from build123d import *

# Parameters (mm, degrees)
SKETCH1_W                = 42
SKETCH1_H                = 120
SKETCH1_R                = 7.5
BOSS_EXTRUDE1_DEPTH      = 10
BOSS_EXTRUDE2_DEPTH      = 6
BOSS_EXTRUDE3_DEPTH      = 6
BOSS_EXTRUDE3_DEPTH_BACK = 42
BOSS_EXTRUDE4_START      = 36
BOSS_EXTRUDE4_DEPTH      = 36
BOSS_EXTRUDE7_START      = -25
SKETCH5_R                = 6
BOSS_EXTRUDE7_DEPTH      = 70
CUT_EXTRUDE1_START       = -70
CUT_EXTRUDE1_DEPTH       = 70


with BuildPart() as part:
    # Sketch1 → Boss-Extrude1 (new body)
    with BuildSketch(Plane(origin=(0, 0, 0), x_dir=(1, 0, 0), z_dir=(0, 1, 0))):
        with Locations((21, 60)):
            Rectangle(SKETCH1_W, SKETCH1_H)
        with Locations(Location((21, 15, 0), (0, 0, 270))):
            Circle(SKETCH1_R, mode=Mode.SUBTRACT)
        with Locations(Location((21, 105, 0), (0, 0, 90))):
            Circle(SKETCH1_R, mode=Mode.SUBTRACT)
    extrude(amount=BOSS_EXTRUDE1_DEPTH)

    # Sketch2 → Boss-Extrude2 (add)
    with BuildSketch(Plane(origin=(42, 0, 0), x_dir=(0, 0, -1), z_dir=(1, 0, 0))):
        with BuildLine():
            Line((90, 25), (90, 86.972243623))
            ThreePointArc((90, 86.972243623), (60, 70), (30, 86.972243623))
            Line((30, 86.972243623), (30, 25))
            ThreePointArc((30, 25), (25.606601718, 14.393398282), (15, 10))
            Line((15, 10), (105, 10))
            ThreePointArc((105, 10), (94.393398282, 14.393398282), (90, 25))
        make_face()
    extrude(amount=-BOSS_EXTRUDE2_DEPTH)

    # Sketch3 → Boss-Extrude3 (add, two sides: drawn at the far end of the back side and taken through both)
    with BuildSketch(Plane(origin=(42, 0, 0), x_dir=(0, 0, -1), z_dir=(1, 0, 0)).offset(-BOSS_EXTRUDE3_DEPTH_BACK)):
        with BuildLine():
            Line((61.5, 134.962476533), (61.5, 139.96784237))
            ThreePointArc((61.5, 139.96784237), (60, 70), (58.5, 139.96784237))
            Line((58.5, 139.96784237), (58.5, 134.962476533))
            ThreePointArc((58.5, 134.962476533), (60, 75), (61.5, 134.962476533))
        make_face()
    extrude(amount=BOSS_EXTRUDE3_DEPTH + BOSS_EXTRUDE3_DEPTH_BACK)

    # Sketch4 → Boss-Extrude4 (add)
    with BuildSketch(Plane.ZY.offset(-36).offset(BOSS_EXTRUDE4_START)):
        with BuildLine():
            Line((-61.5, 10), (-58.5, 10))
            Line((-58.5, 10), (-58.5, 70.03215763))
            ThreePointArc((-58.5, 70.03215763), (-60, 70), (-61.5, 70.03215763))
            Line((-61.5, 70.03215763), (-61.5, 10))
        make_face()
    extrude(amount=-BOSS_EXTRUDE4_DEPTH)

    # Sketch5 → Boss-Extrude7 (add)
    with BuildSketch(Plane.XY.offset(BOSS_EXTRUDE7_START)):
        with BuildLine():
            Line((7, 105), (35, 105))
            Line((35, 105), (35, 147))
            ThreePointArc((35, 147), (21, 161), (7, 147))
            Line((7, 147), (7, 105))
        make_face()
        with Locations((21, 147)):
            Circle(SKETCH5_R, mode=Mode.SUBTRACT)
    extrude(amount=-BOSS_EXTRUDE7_DEPTH)

    # Sketch6 → Cut-Extrude1 (cut)
    with BuildSketch(Plane(origin=(48, 0, 0), x_dir=(0, 0, -1), z_dir=(1, 0, 0)).offset(CUT_EXTRUDE1_START)):
        with BuildLine():
            Line((58.5, 139.96784237), (58.5, 134.962476533))
            ThreePointArc((58.5, 134.962476533), (60, 75), (61.5, 134.962476533))
            Line((61.5, 134.962476533), (61.5, 139.96784237))
            ThreePointArc((61.5, 139.96784237), (60, 140), (58.5, 139.96784237))
        make_face()
    extrude(amount=CUT_EXTRUDE1_DEPTH, mode=Mode.SUBTRACT)


solid = part.part
Geometry: final body of the model. Coordinates: model frame, mm. A direction names the side the tool comes from. Round coordinates to 2 decimals unless told otherwise and drop trailing zeros. Loops run counter-clockwise (first coordinate to the right, second up) from the corner with the lowest first, then second, coordinate; pieces in that order, holes last. Notation, with made-up numbers: (-30.5, 40) -> (-21.5, 40) arc R35 cw to (-21.5, 79) -> close; hole circle Ø1 at (12, -36.5). An arc over 180 degrees is marked (long way). One line per question, with ' | ' between items. Start each with the question number.
1. Mould query, pull axis Z, two halves, no side actions, for faces 1 (the face through (21, 10, -30)), 2 (the face through (24, 138, -58.5)), 3 (the face through (21, 5, 0)). Classes: pulls with the +Z half, pulls with the -Z half, needs draft (parallel to the pull), parting line crosses it, or undercut.
2. Contact query for flat-ended pins moving along their axis: pin 1 (3 mm diameter, centred on x = 39.5, y = 55.5, fed in from +Z); pin 2 (10 mm diameter, centred on y = 29.5, z = -62.5, fed in from +X); pin 3 (8 mm diameter, centred on x = 25.5, y = 107, fed in from -Z). Output: stop coordinate, or through.
3. Section B-B on y = 149.5. Output: boundary loops of the cut face in (x, z), and give its area (3 significant figures).
4. Section C-C on y = 37.5. Output: boundary loops of the cut face in (x, z), and give its area (3 significant figures).
5. Section D-D on y = 122. Output: boundary loops of the cut face in (x, z), and give its area (3 significant figures).
6. Section A-A on x = 21. Output: boundary loops of the cut face in (y, z).
7. Line query: line 1 along X through (y, z) = (7, -15); line 2 along Z through (x, y) = (20, 105); line 3 along Y through (x, z) = (2, -34.5). Output: solid intervals per line, ascending. Write a range as [from, to].
8. Set-up query: faces 4 (the face through (39, 56, -90)), 5 (the face through (18, 40, -58.5)), 6 (the face through (24, 137, -61.5)). Return all of +Z, -Z, +X, -X, +Y, -Y with unobstructed straight access to the full face (end or side cutting, diameter ignored); none if empty.
Returned:
1) face 1: needs draft | face 2: undercut | face 3: pulls with the +Z half
2) pin 1: stops at z = -30 | pin 2: stops at x = 42 | pin 3: stops at z = -95
3) outline: (7.23, -95) -> (15.55, -95) -> (15.55, -25) -> (7.23, -25) -> close; (26.45, -95) -> (34.77, -95) -> (34.77, -25) -> (26.45, -25) -> close | area: 1,160 mm2
4) outline: (0, -61.5) -> (36, -61.5) -> (36, -90) -> (42, -90) -> (42, -30) -> (36, -30) -> (36, -58.5) -> (0, -58.5) -> close | area: 468 mm2
5) outline: (0, -90.59) -> (7, -90.59) -> (7, -95) -> (35, -95) -> (35, -90.59) -> (48, -90.59) -> (48, -84.72) -> (0, -84.72) -> close; (0, -35.28) -> (48, -35.28) -> (48, -29.41) -> (35, -29.41) -> (35, -25) -> (7, -25) -> (7, -29.41) -> (0, -29.41) -> close | area: 811 mm2
6) outline: (0, -120) -> (10, -120) -> (10, -112.5) -> (0, -112.5) -> close; (0, -97.5) -> (10, -97.5) -> (10, -61.5) -> (70.03, -61.5) arc R35 ccw to (105, -95) -> (141, -95) -> (141, -25) -> (105, -25) arc R35 ccw to (70.03, -58.5) -> (10, -58.5) -> (10, -22.5) -> (0, -22.5) -> close; (0, -7.5) -> (10, -7.5) -> (10, 0) -> (0, 0) -> close; (153, -95) -> (161, -95) -> (161, -25) -> (153, -25) -> close; hole (134.96, -61.5) -> (139.97, -61.5) arc R35 ccw to (139.97, -58.5) -> (134.96, -58.5) arc R30 ccw (long way) to start
7) line 1: x = [0, 13.5], [28.5, 42] | line 2: z = [-95, -90], [-30, -25] | line 3: y = [0, 10], [81.03, 89.2], [120.8, 128.97]
8) face 4: -Z, +X, -X | face 5: +Z, -X | face 6: +X, -X
